Model file for the job. Use its own axes, mm. Face numbers are marked on the shaded views. Coordinates: 2 decimals unless noted, no trailing zeros. Loops run counter-clockwise (first coordinate to the right, second up) from the corner with the lowest first, then second, coordinate; pieces in that order, holes last. Notation, with made-up numbers: (-35, 65) -> (1, 65) arc R31 cw to (1, 96) -> close; hole circle Ø7 at (13.25, 77.5). An arc over 180 degrees is marked (long way). Use one line per item in the form item = value.
```python
from build123d import *

# Parameters (mm, degrees)
CUT_EXTRUDE_2_DEPTH = 27.064535292
FILLET_1_R          = 0.6
CHAMFER_1_SIZE      = 0.2
CHAMFER_2_SIZE      = 0.2


with BuildPart() as part:
    # 草图1 → 旋转2 (revolve)
    with BuildSketch(Plane(origin=(0, 0, 0), x_dir=(0, 0, -1), z_dir=(1, 0, 0)), mode=Mode.PRIVATE) as revolve_2_sk:
        Polygon((-16.2, 1), (-18, 1), (-18, 0), (0, 0), (0, 5.6), (-18, 5.6), (-18, 4.6), (-16.2, 4.6), align=None)
    revolve(revolve_2_sk.sketch.rotate(Axis((0, 0, 0), (0, 1, 0)), 180), axis=Axis((0, 0, 0), (0, 1, 0)))

    # 草图2 → 切除-拉伸2 (cut, through all)
    with BuildSketch(Plane(origin=(0, 5.6, 0), x_dir=(1, 0, 0), z_dir=(0, 1, 0))):
        with BuildLine():
            Line((2.5, 1.658312395), (-2.5, 1.658312395))
            ThreePointArc((-2.5, 1.658312395), (-0.866025404, -2.872281323), (3, 0))
            ThreePointArc((3, 0), (2.872281323, 0.866025404), (2.5, 1.658312395))
        make_face()
    extrude(amount=-CUT_EXTRUDE_2_DEPTH, mode=Mode.SUBTRACT)

    # 圆角1
    fillet_1_edges = [part.edges().sort_by_distance(p)[0] for p in [
        (0, 1, 16.2),
        (0, 4.6, 16.2),
    ]]
    fillet(fillet_1_edges, radius=FILLET_1_R)

    # 倒角1
    chamfer_1_edges = [part.edges().sort_by_distance(p)[0] for p in [
        (0, 5.6, -1.658312395),
        (0, 0, 3),
        (0, 0, -1.658312395),
        (0, 5.6, 3),
    ]]
    chamfer(chamfer_1_edges, length=CHAMFER_1_SIZE)

    # 倒角2
    chamfer_2_edges = [part.edges().sort_by_distance(p)[0] for p in [
        (0, 0, 18),
        (0, 5.6, 18),
    ]]
    chamfer(chamfer_2_edges, length=CHAMFER_2_SIZE)


solid = part.part
```
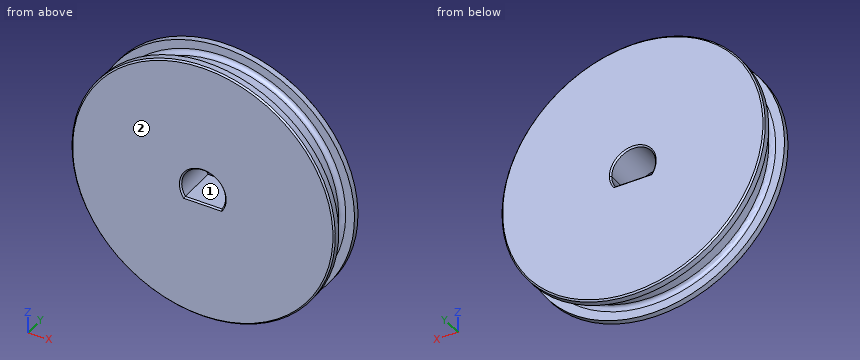
Q1. Band-saw the part on A-A, the plane x = 0. Write the cut outline in (y, z), and give its area (3 significant figures).
Result:
outline = (0, -17.8) -> (0.2, -18) -> (1, -18) -> (1, -16.8) arc R0.6 cw to (1.6, -16.2) -> (4, -16.2) arc R0.6 cw to (4.6, -16.8) -> (4.6, -18) -> (5.4, -18) -> (5.6, -17.8) -> (5.6, -1.86) -> (5.4, -1.66) -> (0.2, -1.66) -> (0, -1.86) -> close; (0, 3.2) -> (0.2, 3) -> (5.4, 3) -> (5.6, 3.2) -> (5.6, 17.8) -> (5.4, 18) -> (4.6, 18) -> (4.6, 16.8) arc R0.6 cw to (4, 16.2) -> (1.6, 16.2) arc R0.6 cw to (1, 16.8) -> (1, 18) -> (0.2, 18) -> (0, 17.8) -> close
area = 163 mm2
Q2. Mould opens along X. For the marked faces 1 and 2 say: released by +X, released by -X, zero draft, split by the parting line, or undercut.
Result:
face_1 = undercut
face_2 = zero draft
Q3. Wall check: line 1 along X through (y, z) = (1.65, 0); line 2 along X through (y, z) = (0.4, -0.5); line 3 along Z through (x, y) = (1.5, 1.8). Give the ranges that are in metal, low to high.
Result:
line_1 = -16.2 to -3, 3 to 16.2
line_2 = -17.99 to -2.96, 2.96 to 17.99
line_3 = -16.13 to -1.66, 2.6 to 16.13
